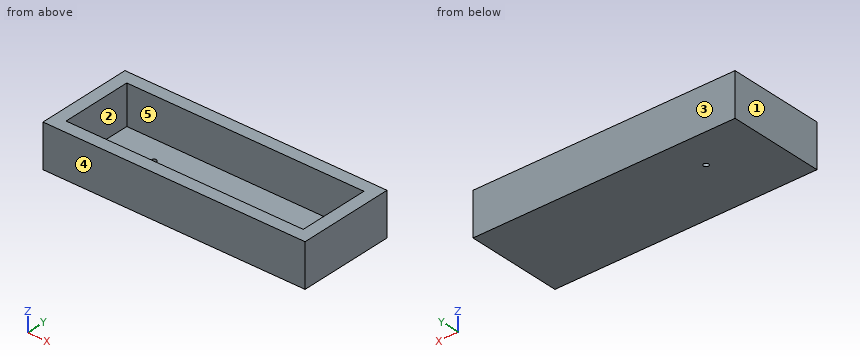
```python
from build123d import *

# Parameters (mm, degrees)
SKETCH_2_W                 = 210.5009
SKETCH_2_H                 = 77.1505
EXTRUDE_1_DEPTH            = 34.5
SHELL_1_T                  = -10
SHELL_1_THICKNESS_2_FACE_W = 190.5009
SHELL_1_THICKNESS_2_FACE_H = 57.1505
SHELL_1_THICKNESS_2_DEPTH  = 7
SKETCH_3_R                 = 2
CUT_EXTRUDE_8_DEPTH        = 3


with BuildPart() as part:
    # 草图2 → 凸台-拉伸1 (new body)
    with BuildSketch(Plane.XY):
        with Locations((95.3455423, 28.832065)):
            Rectangle(SKETCH_2_W, SKETCH_2_H)
    extrude(amount=EXTRUDE_1_DEPTH)

    # 抽壳1
    shell_1_openings = [part.faces().sort_by_distance(p)[0] for p in [
        (95.3455423, 28.832065, 34.5),
    ]]
    offset(amount=SHELL_1_T, openings=shell_1_openings, kind=Kind.INTERSECTION)

    # 抽壳1 thickness 2 face (on inner face of the shell) → 抽壳1 thickness 2 (cut)
    with BuildSketch(Plane(origin=(95.3455423, 28.832065, 10), x_dir=(-1, 0, 0), z_dir=(0, 0, -1))):
        Rectangle(SHELL_1_THICKNESS_2_FACE_W, SHELL_1_THICKNESS_2_FACE_H)
    extrude(amount=SHELL_1_THICKNESS_2_DEPTH, mode=Mode.SUBTRACT)

    # 草图3 → 切除-拉伸8 (cut)
    with BuildSketch(Plane.XY):
        with Locations((38.19575, 38.357)):
            Circle(SKETCH_3_R)
    extrude(amount=CUT_EXTRUDE_8_DEPTH, mode=Mode.SUBTRACT)


solid = part.part
```
Read the model definition and answer for the solid it produces. Units are mm, in the model's axes. Face numbers are marked on the shaded views. A direction names the side the tool comes from. Coordinates: 2 decimals unless noted, no trailing zeros. Write each loop counter-clockwise with the first axis right and the second up, starting at its lowest first coordinate (ties: lowest second). Pieces come first, ordered by that corner, then holes. Notation, with made-up numbers: (10, 40) -> (37, 40) arc R20 cw to (37, 61) -> close; hole circle Ø2 at (49.5, -12). An arc over 180 degrees is marked (long way). Return JSON: item names as keys, results as strings.
1. A cutting plane is placed at C-C (x = 32). Determine the outline of the cut face in (y, z), and give its area (3 significant figures).
Found:
{"outline": "(-9.74, 0) -> (67.41, 0) -> (67.41, 34.5) -> (57.41, 34.5) -> (57.41, 3) -> (0.26, 3) -> (0.26, 34.5) -> (-9.74, 34.5) -> close", "area": "861 mm2"}
2. A cutting plane is placed at B-B (y = 15). Determine the outline of the cut face in (x, z), and give its area (3 significant figures).
Found:
{"outline": "(-9.9, 0) -> (200.6, 0) -> (200.6, 34.5) -> (190.6, 34.5) -> (190.6, 3) -> (0.1, 3) -> (0.1, 34.5) -> (-9.9, 34.5) -> close", "area": "1,260 mm2"}
3. Each of these flat-tipped pins is pushed along its axis until it touches: P1, Ø5, axis at x = 38.2, y = 38.36, coming from the +Z side; P2, Ø6, axis at x = 67.5, y = -0.5, coming from the -Z side. Where does it stop, or does it pass through?
Found:
{"P1": "z = 3", "P2": "z = 0"}
4. A cutting plane is placed at A-A (z = 18). Determine the outline of the cut face in (x, y).
Found:
{"outline": "(-9.9, -9.74) -> (200.6, -9.74) -> (200.6, 67.41) -> (-9.9, 67.41) -> close; hole (0.1, 0.26) -> (190.6, 0.26) -> (190.6, 57.41) -> (0.1, 57.41) -> close"}
5. Determine the mould class of the marked faces 3, 4 and 5 for opening direction Y: pulls with the +Y half, pulls with the -Y half, needs draft (parallel to the pull), parting line crosses it, or undercut.
Found:
{"face 3": "pulls with the +Y half", "face 4": "pulls with the -Y half", "face 5": "undercut"}
6. A tool of negligible diameter and unlimited length cuts with its end or side. For the marked faces 1 and 2, from which of +Z, -Z, +X, -X, +Y, -Y can it reach the whole face along a straight path? Write none if from no direction.
Found:
{"face 1": "+Z, -Z, -X, +Y, -Y", "face 2": "+Z"}
7. Find the intervals of material crossed by line 1 along X through (y, z) = (3.5, 16); line 2 along Y through (x, z) = (156.5, 24.5); line 3 along Z through (x, y) = (146.5, 47), in increasing order. Write a range as from..to.
Found:
{"line 1": "-9.9..0.1, 190.6..200.6", "line 2": "-9.74..0.26, 57.41..67.41", "line 3": "0..3"}
